Here's how the part is built. I have some questions about the finished solid (model axes, mm). A direction names the side the tool comes from. Round coordinates to 2 decimals unless told otherwise and drop trailing zeros. Loops run counter-clockwise (first coordinate to the right, second up) from the corner with the lowest first, then second, coordinate; pieces in that order, holes last. Notation, with made-up numbers: (26, 56) - (69, 56) arc R18 ccw to (69, 72) - close; hole circle Ø4 at (83.25, 29). An arc over 180 degrees is marked (long way). Return JSON: item names as keys, results as strings. Group by question number.
```python
from build123d import *

# Parameters (mm, degrees)
SKETCH2_W           = 10
SKETCH2_H           = 66
BOSS_EXTRUDE1_DEPTH = 1.6
CUT_EXTRUDE1_REACH  = 35.415
SKETCH3_W           = 1
SKETCH3_H           = 5
SKETCH4_W           = 20
SKETCH4_H           = 8
BOSS_EXTRUDE2_DEPTH = 1.6
SKETCH5_W           = 2
SKETCH5_H           = 2
BOSS_EXTRUDE3_DEPTH = 1
SKETCH6_R           = 0.5
BOSS_EXTRUDE4_DEPTH = 2
FILLET1_R           = 0.5


with BuildPart() as part:
    # Sketch2 → Boss-Extrude1 (new body)
    with BuildSketch(Plane(origin=(0, 0, 0), x_dir=(1, 0, 0), z_dir=(0, 1, 0))):
        Rectangle(SKETCH2_W, SKETCH2_H)
    extrude(amount=BOSS_EXTRUDE1_DEPTH)

    # Sketch3 → Cut-Extrude1 (cut, up to next)
    with BuildSketch(Plane(origin=(0, 1.6, 0), x_dir=(1, 0, 0), z_dir=(0, 1, 0)), mode=Mode.PRIVATE) as cut_extrude1_sk1:
        with Locations((1.27, 26.5)):
            Rectangle(SKETCH3_W, SKETCH3_H)
    cut_extrude1_tool1 = extrude(cut_extrude1_sk1.sketch, amount=-CUT_EXTRUDE1_REACH, mode=Mode.PRIVATE) & part.part
    # Sketch3 → Cut-Extrude1 (cut, up to next)
    with BuildSketch(Plane(origin=(0, 1.6, 0), x_dir=(1, 0, 0), z_dir=(0, 1, 0)), mode=Mode.PRIVATE) as cut_extrude1_sk2:
        with Locations((0, 26.5)):
            Rectangle(SKETCH3_W, SKETCH3_H)
    cut_extrude1_tool2 = extrude(cut_extrude1_sk2.sketch, amount=-CUT_EXTRUDE1_REACH, mode=Mode.PRIVATE) & part.part
    # Sketch3 → Cut-Extrude1 (cut, up to next)
    with BuildSketch(Plane(origin=(0, 1.6, 0), x_dir=(1, 0, 0), z_dir=(0, 1, 0)), mode=Mode.PRIVATE) as cut_extrude1_sk3:
        with Locations((-1.27, 26.5)):
            Rectangle(SKETCH3_W, SKETCH3_H)
    cut_extrude1_tool3 = extrude(cut_extrude1_sk3.sketch, amount=-CUT_EXTRUDE1_REACH, mode=Mode.PRIVATE) & part.part
    # Sketch3 → Cut-Extrude1 (cut, up to next)
    with BuildSketch(Plane(origin=(0, 1.6, 0), x_dir=(1, 0, 0), z_dir=(0, 1, 0)), mode=Mode.PRIVATE) as cut_extrude1_sk4:
        with Locations((-1.27, -26.5)):
            Rectangle(SKETCH3_W, SKETCH3_H)
    cut_extrude1_tool4 = extrude(cut_extrude1_sk4.sketch, amount=-CUT_EXTRUDE1_REACH, mode=Mode.PRIVATE) & part.part
    # Sketch3 → Cut-Extrude1 (cut, up to next)
    with BuildSketch(Plane(origin=(0, 1.6, 0), x_dir=(1, 0, 0), z_dir=(0, 1, 0)), mode=Mode.PRIVATE) as cut_extrude1_sk5:
        with Locations((1.27, -26.5)):
            Rectangle(SKETCH3_W, SKETCH3_H)
    cut_extrude1_tool5 = extrude(cut_extrude1_sk5.sketch, amount=-CUT_EXTRUDE1_REACH, mode=Mode.PRIVATE) & part.part
    # Sketch3 → Cut-Extrude1 (cut, up to next)
    with BuildSketch(Plane(origin=(0, 1.6, 0), x_dir=(1, 0, 0), z_dir=(0, 1, 0)), mode=Mode.PRIVATE) as cut_extrude1_sk6:
        with Locations((0, -26.5)):
            Rectangle(SKETCH3_W, SKETCH3_H)
    cut_extrude1_tool6 = extrude(cut_extrude1_sk6.sketch, amount=-CUT_EXTRUDE1_REACH, mode=Mode.PRIVATE) & part.part
    add(cut_extrude1_tool1.solids().sort_by_distance((1.27, 1.6, -26.5))[0], mode=Mode.SUBTRACT)
    add(cut_extrude1_tool2.solids().sort_by_distance((0, 1.6, -26.5))[0], mode=Mode.SUBTRACT)
    add(cut_extrude1_tool3.solids().sort_by_distance((-1.27, 1.6, -26.5))[0], mode=Mode.SUBTRACT)
    add(cut_extrude1_tool4.solids().sort_by_distance((-1.27, 1.6, 26.5))[0], mode=Mode.SUBTRACT)
    add(cut_extrude1_tool5.solids().sort_by_distance((1.27, 1.6, 26.5))[0], mode=Mode.SUBTRACT)
    add(cut_extrude1_tool6.solids().sort_by_distance((0, 1.6, 26.5))[0], mode=Mode.SUBTRACT)

    # Sketch4 → Boss-Extrude2 (add)
    with BuildSketch(Plane.XZ):
        Rectangle(SKETCH4_W, SKETCH4_H)
    extrude(amount=-BOSS_EXTRUDE2_DEPTH)

    # Sketch5 → Boss-Extrude3 (add)
    with BuildSketch(Plane(origin=(0, 1.6, 0), x_dir=(1, 0, 0), z_dir=(0, 1, 0))):
        Rectangle(SKETCH5_W, SKETCH5_H)
        with Locations((4, 0)):
            Rectangle(SKETCH5_W, SKETCH5_H)
    extrude(amount=BOSS_EXTRUDE3_DEPTH)

    # Sketch6 → Boss-Extrude4 (add)
    with BuildSketch(Plane(origin=(0, 2.6, 0), x_dir=(1, 0, 0), z_dir=(0, 1, 0))):
        with Locations(Location((0, 0, 0), (0, 0, 270))):
            Circle(SKETCH6_R)
        with Locations(Location((4, 0, 0), (0, 0, 270))):
            Circle(SKETCH6_R)
    extrude(amount=BOSS_EXTRUDE4_DEPTH)

    # Fillet1
    fillet1_edges = [part.edges().sort_by_distance(p)[0] for p in [
        (0, 4.6, -0.5),
        (4, 4.6, -0.5),
    ]]
    fillet(fillet1_edges, radius=FILLET1_R)


solid = part.part
```
Q1. Please list where these lines run through material, in increasing order: line 1 (X direction, y = 0.7, z = -24.5); line 2 (Y direction, x = 3, z = -22); line 3 (X direction, y = 0.2, z = 10).
Q2. For faces 1 (the flat face through (0.5, 1, 27)), 2 (the flat face through (3.5, 2.6, -0.5)), 3 (the flat face through (-5, 1, 19)), which set-ups out of +Z, -Z, +X, -X, +Y, -Y let a thin tool reach every point of the face, with its end or its side?
Q3. Imagine slicing it at B-B, the plane y = 0.7. Give the number of separate pieces and of enclosed holes in the cut face, and give its area (3 significant figures).
Q4. Imagine slicing it at C-C, the plane x = -3.5. List the corners of the cut face in (y, z) for me, and give its area (3 significant figures).
Q5. Will these pins go through, and if not, where does the flat tip stop? pin 1 Ø1.8 at (y, z) = (1, 27) entering from +X; pin 2 Ø0.5 at (y, z) = (0.5, 26.5) entering from -X; pin 3 Ø8 at (x, z) = (-1.5, 7) entering from +Y.
Q6. Imagine slicing it at D-D, the plane z = -15. List the corners of the cut face in (x, y) for me, and give its area (3 significant figures).
Q7. If we mould it in two halves opening along Z, with no side actions, what happens to faces 4 (the flat face through (-0.5, 1, -26)), 5 (the flat face through (-8, 1, 4)), 6 (the flat face through (0, 1, -33)), 7 (the flat face through (-10, 1, 0))? For each: +Z half, -Z half, draft (parallel to the pull), parting line (faces both ways), or undercut.
Q8. Imagine slicing it at A-A, the plane z = 26.5. List the corners of the cut face in (x, y) for me, and give its area (3 significant figures).
Output values:
{
 "1": {"line 1": "x = -5 to -1.77, -0.77 to -0.5, 0.5 to 0.77, 1.77 to 5", "line 2": "y = 0 to 1.6", "line 3": "x = -5 to 5"},
 "2": {"face 1": "+Y, -Y", "face 2": "+Y", "face 3": "+Z, -X, +Y, -Y"},
 "3": {"separate pieces": "1", "enclosed holes": "6", "area": "710 mm^2"},
 "4": {"outline": "(0, -33) - (1.6, -33) - (1.6, 33) - (0, 33) - close", "area": "106 mm^2"},
 "5": {"pin 1": "stops at x = 5", "pin 2": "stops at x = -5", "pin 3": "stops at y = 1.6"},
 "6": {"outline": "(-5, 0) - (5, 0) - (5, 1.6) - (-5, 1.6) - close", "area": "16.0 mm^2"},
 "7": {"face 4": "undercut", "face 5": "+Z half", "face 6": "-Z half", "face 7": "draft"},
 "8": {"outline": "(-5, 0) - (-1.77, 0) - (-1.77, 1.6) - (-5, 1.6) - close; (-0.77, 0) - (-0.5, 0) - (-0.5, 1.6) - (-0.77, 1.6) - close; (0.5, 0) - (0.77, 0) - (0.77, 1.6) - (0.5, 1.6) - close; (1.77, 0) - (5, 0) - (5, 1.6) - (1.77, 1.6) - close", "area": "11.2 mm^2"}
}
